For this review, take the finished solid that the model builds, in its own axes (mm). A direction names the side the tool comes from. Coordinates: 2 decimals unless noted, no trailing zeros. Write each loop counter-clockwise with the first axis right and the second up, starting at its lowest first coordinate (ties: lowest second). Pieces come first, ordered by that corner, then holes. Notation, with made-up numbers: (-9, -2) -> (10, -2) arc R16 ccw to (10, 9) -> close; hole circle Ø11 at (35, 3.25). An arc over 180 degrees is marked (long way). Put each result on its own line as item: value. Start each with the question number.
Item 1: Consider section D-D on y = -1.25. Give the boundary of the cut face in (x, z).
Item 2: Insertion check: P1, Ø1, axis at y = -0.5, z = -3.5, coming from the +X side; P2, Ø6, axis at x = -4, z = 3.5, coming from the +Y side; P3, Ø6, axis at x = 6, z = -0.5, coming from the -Y side. Each pin has a flat end and moves straight along its axis. Give the tip position at first contact, or say it passes through.
Item 3: Consider section C-C on y = 0.25. Give the boundary of the cut face in (x, z), and give its area (3 significant figures).
Item 4: For faces 1 (the flat face through (0, -4.9, 0)), 2 (the cylindrical face through (-0.867, -2.12, -3.905)), 3 (the cylindrical face through (-9.49, 0.2, 0.24)), list the 3-axis set-ups (+Z, -Z, +X, -X, +Y, -Y) from which the entire face can be reached by the end or side of a thin tool; tool diameter is ignored.
Item 5: To check wall thickness, follow L1, parallel to Y at x = 6.5, z = 1.5; L2, parallel to Y at x = 2.5, z = -2.75; L3, parallel to X at y = -0.25, z = -0.25. State the ranges of each line that lie inside material, in increasing order.
Item 6: Consider section A-A on z = 0. Give the boundary of the cut face in (x, y).
Item 7: Consider section B-B on x = 0. Give the boundary of the cut face in (y, z).
```python
from build123d import *

# Parameters (mm, degrees)
F2_R        = 2.5
F3_DEPTH    = 1.5
F4_R        = 1
F5_S5_R     = 2.5
F5_T6_DEPTH = 16


# Not quite as in the source:
# - a fillet or chamfer that OpenCascade refuses, or shapes differently, is made with other operations: its cross-section is extruded or revolved along the edge and cut away or added


with BuildPart() as f1:
    # F0 (on Top) → F1 (revolve)
    with BuildSketch(Plane.XY):
        Polygon((0, 0), (0, -4.9), (2.6, -4.9), (2.6, -2.8), (2.6, -2.5), (4, -2.5), (4, -1.75), (10, -1.75), (10, 0), align=None)
    revolve(axis=Axis((0, -2.45, 0), (0, -1, 0)))

    # F2 (on face) → F3 (join)
    with BuildSketch(Plane(origin=(0, 0, 0), x_dir=(-1, 0, 0), z_dir=(0, 1, 0))):
        with Locations((7, 0)):
            Circle(F2_R)
    extrude(amount=F3_DEPTH)

    # F4
    f4_edges = [f1.edges().sort_by_distance(p)[0] for p in [
        (-4.5, 1.5, 0),
    ]]
    fillet(f4_edges, radius=F4_R)

    # F5: chamfer of 0.75 on 1 edges, made by hand


with BuildPart() as f5_tool2:
    # F5_s3 → F5_t4 (revolve)
    with BuildSketch(Plane.XY):
        Polygon((9.25, 0), (10, -0.75), (10, 0), align=None)
    revolve(axis=Axis((0, 0, 0), (0, -1, 0)))

    # F5_s5 → F5_t6 (cut, symmetric)
    with BuildSketch(Plane.XZ.offset(0.4)):
        with Locations((-7, 0)):
            Circle(F5_S5_R)
    extrude(amount=F5_T6_DEPTH, both=True, mode=Mode.SUBTRACT)


with BuildPart() as f1_1:
    add(f1.part)

    # F5_t1: cut F5_tool2
    add(f5_tool2.part, mode=Mode.SUBTRACT)


solid = f1_1.part
```
Return value:
1. outline: circle Ø20 at (0, 0)
2. P1: x = 9.52
2. P2: y = 1.49
2. P3: y = -2.5
3. outline: circle Ø5 at (-7, 0)
3. area: 19.6 mm^2
4. face 1: +Z, -Z, +X, -X, -Y
4. face 2: -Y
4. face 3: +Y
5. L1: -1.75 to 0
5. L2: -2.5 to 0
5. L3: -9.5 to 9.5
6. outline: (-10, -1.75) -> (-4, -1.75) -> (-4, -2.5) -> (-2.6, -2.5) -> (-2.6, -4.9) -> (2.6, -4.9) -> (2.6, -2.5) -> (4, -2.5) -> (4, -1.75) -> (10, -1.75) -> (10, -0.75) -> (9.25, 0) -> (-4.5, 0) -> (-4.5, 0.5) arc R1 ccw to (-5.5, 1.5) -> (-8.5, 1.5) arc R1 ccw to (-9.5, 0.5) -> (-9.5, -0.25) -> (-10, -0.75) -> close
7. outline: (-4.9, -2.6) -> (-2.5, -2.6) -> (-2.5, -4) -> (-1.75, -4) -> (-1.75, -10) -> (-0.75, -10) -> (0, -9.25) -> (0, 9.25) -> (-0.75, 10) -> (-1.75, 10) -> (-1.75, 4) -> (-2.5, 4) -> (-2.5, 2.6) -> (-4.9, 2.6) -> close
